Geometry: final body of the model. Coordinates: model frame, mm. Round coordinates to 2 decimals unless told otherwise and drop trailing zeros. Order: outer loops, then holes, each group sorted by start corner. A loop starts at its lowest first (then second) coordinate and runs counter-clockwise, first axis right, second up. Notation, with made-up numbers: M 53.25,13.5 L 69.25,13.5 A26 ccw 69.25,35.5 Z; hole C 56,34 d7. An arc over 180 degrees is marked long. Return JSON: item names as keys, results as strings. Group by question number.
Q1. Cut plane B-B on z = 1.65. Count the separate pieces of the cut face and the enclosed holes in it, and give its area (3 significant figures).
Q2. Cut plane C-C on x = 299.5. Output: boundary loops of the cut face in (y, z), and give its area (3 significant figures).
Q3. Cut plane A-A on x = 136.5. Output: boundary loops of the cut face in (y, z).
Q4. Contact query for flat-ended pins moving along their axis: pin 1 (5.5 mm diameter, centred on x = 121, y = 90, fed in from -Z); pin 2 (2 mm diameter, centred on y = 40, z = 3, fed in from +X). Output: stop coordinate, or through.
Q5. Ray query, probe 1 along X at (y, z) = (211.5, 3.3); probe 2 along X at (y, z) = (290.5, 2.35); probe 3 along Y at (x, z) = (219, 3.7). Return the intervals inside material, ascending.
Q6. Cut plane D-D on y = 242. Output: boundary loops of the cut face in (x, z), and give its area (3 significant figures).
```python
from build123d import *

# Parameters (mm, degrees)
F0_W      = 320
F0_H      = 420
F1_DEPTH  = 4
F3_DEPTH  = 4
F4_R      = 3
F5_DEPTH  = 25
F6_R      = 3
F7_DEPTH  = 25
F8_R      = 3
F9_DEPTH  = 25
F11_DEPTH = 25


with BuildPart() as f1:
    # F0 (on Top) → F1 (new body)
    with BuildSketch(Plane.XY):
        with Locations((160, 210)):
            Rectangle(F0_W, F0_H)
    extrude(amount=F1_DEPTH)

    # F2 (on face) → F3 (cut, through all)
    with BuildSketch(Plane.XY.offset(4)):
        Polygon((320, 420), (290, 420), (320, 360), align=None)
        Polygon((320, 60), (290, 0), (320, 0), align=None)
        with BuildLine():
            Line((113, 360), (213, 360))
            ThreePointArc((213, 360), (216.535534, 361.464466), (218, 365))
            Line((218, 365), (218, 403))
            ThreePointArc((218, 403), (216.535534, 406.535534), (213, 408))
            Line((213, 408), (113, 408))
            ThreePointArc((113, 408), (109.464466, 406.535534), (108, 403))
            Line((108, 403), (108, 365))
            ThreePointArc((108, 365), (109.464466, 361.464466), (113, 360))
        make_face()
        with BuildLine():
            Line((113, 12), (213, 12))
            ThreePointArc((213, 12), (216.535534, 13.464466), (218, 17))
            Line((218, 17), (218, 55))
            ThreePointArc((218, 55), (216.535534, 58.535534), (213, 60))
            Line((213, 60), (113, 60))
            ThreePointArc((113, 60), (109.464466, 58.535534), (108, 55))
            Line((108, 55), (108, 17))
            ThreePointArc((108, 17), (109.464466, 13.464466), (113, 12))
        make_face()
        Polygon((0, 420), (0, 210), (50, 420), align=None)
        Polygon((50, 0), (0, 210), (0, 0), align=None)
    extrude(amount=-F3_DEPTH, mode=Mode.SUBTRACT)

    # F4 (on face) → F5 (cut)
    with BuildSketch(Plane.XY.offset(4)):
        with Locations((67, 6)):
            Circle(F4_R)
        with Locations((97, 6)):
            Circle(F4_R)
        with Locations((127, 6)):
            Circle(F4_R)
        with Locations((157, 6)):
            Circle(F4_R)
        with Locations((187, 6)):
            Circle(F4_R)
        with Locations((217, 6)):
            Circle(F4_R)
        with Locations((247, 6)):
            Circle(F4_R)
        with Locations((277, 6)):
            Circle(F4_R)
        with Locations((64, 66)):
            Circle(F4_R)
        with Locations((94, 66)):
            Circle(F4_R)
        with Locations((124, 66)):
            Circle(F4_R)
        with Locations((220, 66)):
            Circle(F4_R)
        with Locations((250, 66)):
            Circle(F4_R)
        with Locations((280, 66)):
            Circle(F4_R)
        with Locations((310, 66)):
            Circle(F4_R)
        with Locations((67, 414)):
            Circle(F4_R)
        with Locations((64, 354)):
            Circle(F4_R)
        with Locations((97, 414)):
            Circle(F4_R)
        with Locations((310, 354)):
            Circle(F4_R)
        with Locations((277, 414)):
            Circle(F4_R)
        with Locations((94, 354)):
            Circle(F4_R)
        with Locations((220, 354)):
            Circle(F4_R)
        with Locations((280, 354)):
            Circle(F4_R)
        with Locations((124, 354)):
            Circle(F4_R)
        with Locations((127, 414)):
            Circle(F4_R)
        with Locations((250, 354)):
            Circle(F4_R)
        with Locations((157, 414)):
            Circle(F4_R)
        with Locations((187, 414)):
            Circle(F4_R)
        with Locations((217, 414)):
            Circle(F4_R)
        with Locations((247, 414)):
            Circle(F4_R)
    extrude(amount=-F5_DEPTH, mode=Mode.SUBTRACT)

    # F6 (on face) → F7 (cut)
    with BuildSketch(Plane.XY.offset(4)):
        with Locations((121, 90)):
            Circle(F6_R)
        with Locations((121, 130)):
            Circle(F6_R)
        with Locations((121, 170)):
            Circle(F6_R)
        with Locations((206, 90)):
            Circle(F6_R)
        with Locations((206, 130)):
            Circle(F6_R)
        with Locations((206, 170)):
            Circle(F6_R)
        with Locations((291.000009, 80.000006)):
            Circle(F6_R)
        with Locations((291.000009, 120.000006)):
            Circle(F6_R)
        with Locations((291.000009, 160.000006)):
            Circle(F6_R)
        with Locations((121, 330)):
            Circle(F6_R)
        with Locations((121, 290)):
            Circle(F6_R)
        with Locations((206, 330)):
            Circle(F6_R)
        with Locations((206, 250)):
            Circle(F6_R)
        with Locations((291.000009, 339.99999)):
            Circle(F6_R)
        with Locations((121, 250)):
            Circle(F6_R)
        with Locations((206, 290)):
            Circle(F6_R)
        with Locations((291.000009, 299.99999)):
            Circle(F6_R)
        with Locations((291.000009, 259.99999)):
            Circle(F6_R)
    extrude(amount=-F7_DEPTH, mode=Mode.SUBTRACT)

    # F8 (on face) → F9 (cut)
    with BuildSketch(Plane.XY.offset(4)):
        with Locations((15, 210)):
            Circle(F8_R)
        with Locations((45, 210)):
            Circle(F8_R)
    extrude(amount=-F9_DEPTH, mode=Mode.SUBTRACT)

    # F10 (on face) → F11 (cut)
    with BuildSketch(Plane.XY.offset(4)):
        with BuildLine():
            ThreePointArc((192.858117, 288.5), (185, 282), (177.141883, 288.5))
            Line((177.141883, 288.5), (169.583592, 288.5))
            ThreePointArc((169.583592, 288.5), (183, 278.5), (196.416408, 288.5))
            Line((196.416408, 288.5), (192.858117, 288.5))
        make_face()
        with BuildLine():
            ThreePointArc((193, 130), (185, 122), (177, 130))
            Line((177, 130), (169.225023, 130))
            ThreePointArc((169.225023, 130), (183, 113.5), (196.774977, 130))
            Line((196.774977, 130), (193, 130))
        make_face()
        with BuildLine():
            ThreePointArc((195.399597, 134), (183, 141.5), (170.600403, 134))
            Line((170.600403, 134), (178.071797, 134))
            ThreePointArc((178.071797, 134), (185, 138), (191.928203, 134))
            Line((191.928203, 134), (195.399597, 134))
        make_face()
        with BuildLine():
            ThreePointArc((197, 292.5), (183, 306.5), (169, 292.5))
            Line((169, 292.5), (177.400658, 292.5))
            ThreePointArc((177.400658, 292.5), (185, 298), (192.599342, 292.5))
            Line((192.599342, 292.5), (197, 292.5))
        make_face()
    extrude(amount=-F11_DEPTH, mode=Mode.SUBTRACT)


solid = f1.part
```
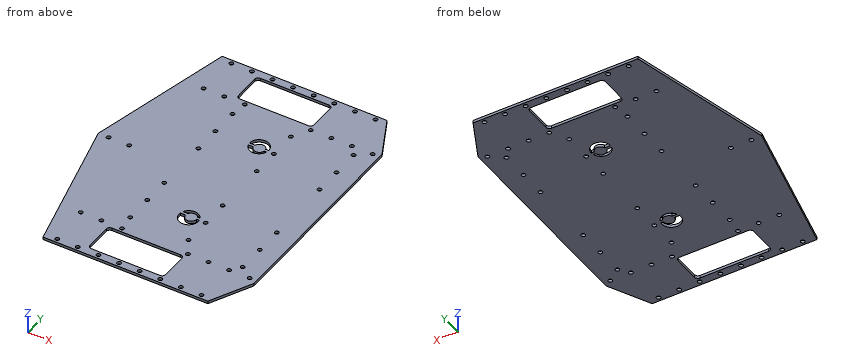
Result sheet:
{
 "1": {"separate pieces": "1", "enclosed holes": "56", "area": "109,000 mm²"},
 "2": {"outline": "M 19,0 L 401,0 L 401,4 L 19,4 Z", "area": "1,530 mm²"},
 "3": {"outline": "M 0,0 L 12,0 L 12,4 L 0,4 Z; M 60,0 L 360,0 L 360,4 L 60,4 Z; M 408,0 L 420,0 L 420,4 L 408,4 Z"},
 "4": {"pin 1": "passes through", "pin 2": "stops at x = 310.5"},
 "5": {"probe 1": "x = 0.36 to 12.4, 17.6 to 42.4, 47.6 to 320", "probe 2": "x = 19.17 to 118.04, 123.96 to 203.04, 208.96 to 320", "probe 3": "y = 0 to 3.76, 8.24 to 63.17, 68.83 to 351.17, 356.83 to 411.76, 416.24 to 420"},
 "6": {"outline": "M 7.62,0 L 320,0 L 320,4 L 7.62,4 Z", "area": "1,250 mm²"}
}
